Can you work these out from the model? Positions are in its coordinate system, mm. A direction names the side the tool comes from. Give positions to 0.01 mm unless a question says otherwise; leave off trailing zeros. Order: outer loops, then holes, each group sorted by start corner. A loop starts at its lowest first (then second) coordinate and runs counter-clockwise, first axis right, second up.
Item 1: I want a section at B-B, the plane z = 134.5. Write out the boundary of the cut face in (x, y) (3 decimals), then the cut area to 3 significant figures.
Item 2: I want a section at A-A, the plane y = 6.5. Write out the boundary of the cut face in (x, z).
Item 3: If I drill on line 1 along Z through (x, y) = (-178.5, 6.75); line 2 along X through (y, z) = (-7.25, 278.5), over which ranges is the centre line in solid material (lowest first)?
Item 4: Which directions (+Z, -Z, +X, -X, +Y, -Y) give clear straight access to the entire face, cutting with the end or side of a thin tool? Please do faces 1 (the flat face through (-115, 3.175, -64)), 2 (the flat face through (-185, 3.175, 310)), 3 (the flat face through (-177, 0, -438.15)).
Item 5: I'm going to push flat-ended pins straight in: pin 1 Ø9.5 at (x, z) = (-193, 310.5) entering from +Y (3 decimals); pin 2 Ø9.5 at (x, z) = (-112.5, 75) entering from -Y (3 decimals); pin 3 Ø10 at (y, z) = (-4.5, -88.5) entering from +X. Where does each tip first touch, or does it pass through?
Item 6: If we mould it in two halves opening along X, with no side actions, what happens to faces 4 (the flat face through (-247.904, 0, 6)), 5 (the flat face through (-115, 3.175, 379))? For each: +X half, -X half, draft (parallel to the pull), parting line (faces both ways), or undercut.
```python
from build123d import *

# Parameters (mm, degrees)
F0_W     = 142.875
F0_H     = 438.15
F1_DEPTH = 9.525
F2_W     = 142.875
F2_H     = 19.05
F3_DEPTH = 6.35
F4_W     = 19.05
F4_H     = 876.3
F5_DEPTH = 12.7


# Not quite as in the source:
# - a feature names something its author has since deleted; it is built from what else it names


with BuildPart() as f1:
    # F0 (on Front) → F1 (new body, symmetric)
    with BuildSketch(Plane.XZ):
        with Locations((-176.4664953259, 219.075)):
            Rectangle(F0_W, F0_H)
        with Locations((-176.4664953259, -219.075)):
            Rectangle(F0_W, F0_H)
    extrude(amount=F1_DEPTH, both=True)

    # F2 (on face) → F3 (cut)
    with BuildSketch(Plane(origin=(0, 9.525, 0), x_dir=(-1, 0, 0), z_dir=(0, 1, 0))):
        with Locations((176.4664953259, 309.5625)):
            Rectangle(F2_W, F2_H)
    extrude(amount=-F3_DEPTH, mode=Mode.SUBTRACT)

    # F4 (on face) → F5 (cut)
    with BuildSketch(Plane.XZ.offset(9.525)):
        with Locations((-114.5539953259, 0)):
            Rectangle(F4_W, F4_H)
    extrude(amount=-F5_DEPTH, mode=Mode.SUBTRACT)


solid = f1.part
```
Results list:
1. outline: (-247.904, -9.525) - (-124.079, -9.525) - (-124.079, 3.175) - (-105.029, 3.175) - (-105.029, 9.525) - (-247.904, 9.525) - close
1. area: 2,480 mm2
2. outline: (-247.9, -438.15) - (-105.03, -438.15) - (-105.03, 300.04) - (-247.9, 300.04) - close; (-247.9, 319.09) - (-105.03, 319.09) - (-105.03, 438.15) - (-247.9, 438.15) - close
3. line 1: z = -438.15 to 300.04, 319.09 to 438.15
3. line 2: x = -247.9 to -124.08
4. face 1: +Z, -Z, +X, -Y
4. face 2: +X, -X, +Y
4. face 3: -Z, +X, -X, +Y, -Y
5. pin 1: stops at y = 3.175
5. pin 2: stops at y = 3.175
5. pin 3: stops at x = -124.08
6. face 4: -X half
6. face 5: draft
